from build123d import *

# Parameters (mm, degrees)
F1_DEPTH  = 38.862
F2_DEPTH  = 23.622
F3_DEPTH  = 23.368
F5_DEPTH  = 79.248
F7_DEPTH  = 75.692
F8_W      = 6.6682146308
F8_H      = 6.8875169381
F9_DEPTH  = 99.314
F11_DEPTH = 23.622


with BuildPart() as f1:
    # F0 (on Right) → F1 (new body)
    with BuildSketch(Plane.YZ):
        Polygon((31.3382074237, 23.87672849), (-22.4620722006, 23.87672849), (-45.3531080303, -22.2696410492), (31.3382074237, -22.2696410492), align=None)
    extrude(amount=F1_DEPTH)

    # F2 (add): faces of the model
    f2_faces = [f1.faces().sort_by_distance(p)[0] for p in [
        (19.431, 4.4380676116, 23.87672849),
        (19.431, -33.9075901154, 0.8035437204),
    ]]
    extrude(f2_faces, amount=F2_DEPTH, dir=(0, 0, 1))

    # F3 (add): a face of the model
    f3_faces = [f1.faces().sort_by_distance(p)[0] for p in [
        (19.431, -33.9075901154, 24.4255437204),
    ]]
    extrude(f3_faces, amount=F3_DEPTH)

    # F4 (on face) → F5 (cut)
    with BuildSketch(Plane.YZ.offset(38.862)):
        Polygon((14.3489968032, 28.0092395842), (-30.6494552642, 27.779655531), (-30.6494552642, -9.4129415229), (14.3489968032, -9.4129415229), align=None)
    extrude(amount=-F5_DEPTH, mode=Mode.SUBTRACT)

    # F6 (on face) → F7 (cut)
    with BuildSketch(Plane.YZ.offset(38.862)):
        Polygon((-28.0031748116, 38.1083898246), (-38.2806286216, 44.1071428359), (-51.7797023058, 17.9995857179), (-30.6494552642, 9.1833570041), (-30.6494552642, 27.779655531), align=None)
    extrude(amount=-F7_DEPTH, mode=Mode.SUBTRACT)

    # F8 (on face) → F9 (cut)
    with BuildSketch(Plane.YZ.offset(38.862)):
        with Locations((-42.0190007149, -18.8258825801)):
            Rectangle(F8_W, F8_H)
    extrude(amount=-F9_DEPTH, mode=Mode.SUBTRACT)

    # F10 (on face) → F11 (join)
    with BuildSketch(Plane(origin=(0, 31.3382074237, 0), x_dir=(-1, 0, 0), z_dir=(0, 1, 0))):
        Polygon((-12.3405372724, 25.5852285773), (-30.064733699, 26.704614982), (-30.064733699, -5.189940799), (-12.3405372724, -5.189940799), align=None)
    extrude(amount=F11_DEPTH)


solid = f1.part
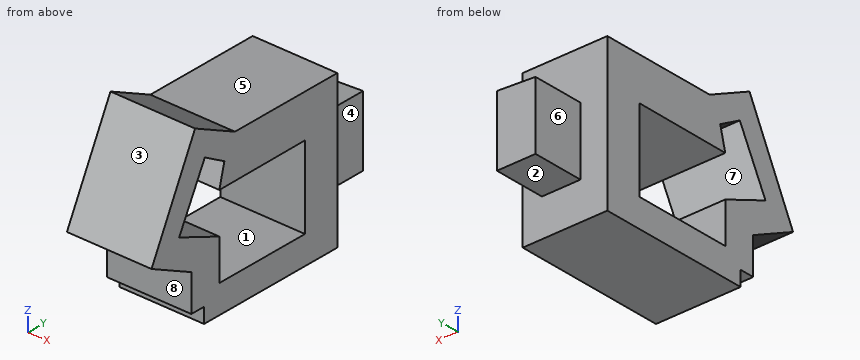
Work out the finished part from the listing and answer in its coordinate system (mm). Face numbers are marked on the shaded views. A direction names the side the tool comes from. Give positions to 0.01 mm unless a question says otherwise; leave off trailing zeros. Write each loop counter-clockwise with the first axis right and the second up, starting at its lowest first coordinate (ties: lowest second). Pieces come first, ordered by that corner, then holes. Notation, with made-up numbers: (53, 17.25) - (68, 17.25) arc R35 cw to (68, 51.25) - close; hole circle Ø10 at (-4.5, 81). An arc over 180 degrees is marked (long way). One line per item, written item: value. Start each with the question number.
1. Find section A-A (x = 35). Write down the section's boundary in (y, z), then the cut area to 3 significant figures.
2. Find section D-D (y = 23). Write down the section's boundary in (x, z), then the cut area to 3 significant figures.
3. Consider probe 1 along Y at (x, z) = (23, -5); probe 2 along Y at (x, z) = (6.5, -4.5); probe 3 along Z at (x, y) = (17.5, 13.5). Determine where each line is inside the solid, lowest interval first.
4. Given pin 1 (1.5 mm diameter, centred on x = 34.5, z = 7.5, fed in from +Y); pin 2 (12 mm diameter, centred on y = 42.5, z = 10.5, fed in from -X); pin 3 (3 mm diameter, centred on x = 28, z = 35.5, fed in from -Y), each flat-ended and moving along its own axis, determine where each tip first touches the part or whether it passes through.
5. Find section C-C (z = 32). Write down the section's boundary in (x, y).
6. For a pull along Y with two mould halves and no side action, classify the marked faces 1, 2 and 3 as +Y half, -Y half, draft (parallel to the pull), parting line (faces both ways), or undercut.
7. Find section B-B (y = -2.5). Write down the section's boundary in (x, z).
8. For the marked faces 4, 5, 6, 7 and 8, determine the directions among +Z, -Z, +X, -X, +Y, -Y from which every point of the face is accessible in a straight line to the end or side of a thin tool.
Geometry results:
1. outline: (-66.29, 11.74) - (-45.35, 1.35) - (-45.35, -15.38) - (-38.68, -15.38) - (-38.68, -22.27) - (31.34, -22.27) - (31.34, 47.5) - (-22.46, 47.5) - (-43.4, 57.88) - close; hole (-51.78, 18) - (-30.65, 9.18) - (-30.65, -9.41) - (14.35, -9.41) - (14.35, 28.01) - (-30.65, 27.78) - (-28, 38.11) - (-38.28, 44.11) - close
1. area: 3,830 mm2
2. outline: (0, -22.27) - (38.86, -22.27) - (38.86, 47.5) - (0, 47.5) - close
2. area: 2,710 mm2
3. probe 1: -45.35 to -30.65, 14.35 to 54.96
3. probe 2: -45.35 to -30.65, 14.35 to 31.34
3. probe 3: -22.27 to -9.41, 28 to 47.5
4. pin 1: y = 31.34
4. pin 2: x = 12.34
4. pin 3: y = -55.24
5. outline: (0, -56.24) - (38.86, -56.24) - (38.86, -44.54) - (0, -44.54) - close; (0, -29.57) - (38.86, -29.57) - (38.86, 31.34) - (0, 31.34) - close
6. face 1: undercut
6. face 2: draft
6. face 3: -Y half
7. outline: (0, -22.27) - (38.86, -22.27) - (38.86, -9.41) - (0, -9.41) - close; (0, 27.92) - (38.86, 27.92) - (38.86, 47.5) - (0, 47.5) - close
8. face 4: +Z, -Z, +X, +Y
8. face 5: +Z, +X, -X, +Y
8. face 6: +Z, -Z, -X, +Y
8. face 7: +X, -X
8. face 8: -Z, +X, -X, -Y
